```python
from build123d import *

# Parameters (mm, degrees)
SKETCH_1_R          = 17.5
EXTRUDE_1_DEPTH     = 9
SKETCH_2_R          = 1.3
CUT_EXTRUDE_1_DEPTH = 8
SKETCH_3_R          = 1.65
CUT_EXTRUDE_2_DEPTH = 9
SKETCH_4_R          = 7
CUT_EXTRUDE_3_DEPTH = 9
CHAMFER_1_SIZE      = 0.4
CHAMFER_1_SIZE2     = 1.098990968
SKETCH_5_R          = 3.2
CUT_EXTRUDE_4_DEPTH = 5


with BuildPart() as part:
    # 草图1 → 凸台-拉伸1 (new body)
    with BuildSketch(Plane.XY):
        Circle(SKETCH_1_R)
    extrude(amount=-EXTRUDE_1_DEPTH)

    # 草图2 → 切除-拉伸1 (cut)
    with BuildSketch(Plane.XY):
        with Locations((12.5, 0)):
            Circle(SKETCH_2_R)
        with Locations((0, -12.5)):
            Circle(SKETCH_2_R)
        with Locations((-12.5, 0)):
            Circle(SKETCH_2_R)
        with Locations((0, 12.5)):
            Circle(SKETCH_2_R)
    extrude(amount=-CUT_EXTRUDE_1_DEPTH, mode=Mode.SUBTRACT)

    # 草图3 → 切除-拉伸2 (cut)
    with BuildSketch(Plane.XY):
        with Locations((6.75, -11.691342951)):
            Circle(SKETCH_3_R)
        with Locations((-6.75, -11.691342951)):
            Circle(SKETCH_3_R)
        with Locations((-6.75, 11.691342951)):
            Circle(SKETCH_3_R)
        with Locations((6.75, 11.691342951)):
            Circle(SKETCH_3_R)
    extrude(amount=-CUT_EXTRUDE_2_DEPTH, mode=Mode.SUBTRACT)

    # 草图4 → 切除-拉伸3 (cut)
    with BuildSketch(Plane.XY):
        Circle(SKETCH_4_R)
    extrude(amount=-CUT_EXTRUDE_3_DEPTH, mode=Mode.SUBTRACT)

    # 倒角1
    chamfer_1_edges = [part.edges().sort_by_distance(p)[0] for p in [
        (-1.3, -12.5, 0),
        (-13.8, 0, 0),
        (-1.3, 12.5, 0),
        (11.2, 0, 0),
    ]]
    chamfer_1_side = [part.faces().sort_by_distance(p)[0] for p in [
        (-17.005025253, 0, 0),
    ]]
    chamfer(chamfer_1_edges, length=CHAMFER_1_SIZE, length2=CHAMFER_1_SIZE2, reference=chamfer_1_side[0])

    # 草图5 → 切除-拉伸4 (cut)
    with BuildSketch(Plane.XY):
        with Locations((-6.75, 11.691342951)):
            Circle(SKETCH_5_R)
        with Locations((6.75, 11.691342951)):
            Circle(SKETCH_5_R)
        with Locations((6.75, -11.691342951)):
            Circle(SKETCH_5_R)
        with Locations((-6.75, -11.691342951)):
            Circle(SKETCH_5_R)
    extrude(amount=-CUT_EXTRUDE_4_DEPTH, mode=Mode.SUBTRACT)


solid = part.part
```
Here's how the part is built. I have some questions about the finished solid (model axes, mm). A direction names the side the tool comes from. Give positions to 0.01 mm unless a question says otherwise; leave off trailing zeros. Loops run counter-clockwise (first coordinate to the right, second up) from the corner with the lowest first, then second, coordinate; pieces in that order, holes last. Notation, with made-up numbers: M 64,42 L 72,42 A10 ccw 72,56 Z; hole C 12,45 d6. An arc over 180 degrees is marked long. Put each result on its own line as item: value. Start each with the question number.
(1) I want a section at B-B on y = -12.5. Please give me the cut outline in (x, z), then the cut area to 3 significant figures.
(2) For faces 4 (the flat face through (8, 10, -5)), 5 (the cylindrical face through (6.39, 10.08, -6.97)), which set-ups out of +Z, -Z, +X, -X, +Y, -Y let a thin tool reach every point of the face, with its end or its side?
(3) I want a section at C-C on y = -5. Please give me the cut outline in (x, z).
(4) Will these pins go through, and if not, where does the flat tip stop? pin 1 Ø3 at (x, y) = (6.5, 11.5) entering from +Z; pin 2 Ø5 at (x, z) = (-12.5, -1.5) entering from -Y; pin 3 Ø2 at (x, z) = (13.5, -3) entering from +Y.
(5) I need wall thicknesses on line 1 along X through (y, z) = (-10, -1.25); line 2 along Y through (x, z) = (-0.5, -1.75); line 3 along Y through (x, z) = (-1, -5.5). Which ranges of each line are inside material? Lowest first, please. Write a range as [from, to].
(6) I want a section at A-A on x = 0. Please give me the cut outline in (y, z), then the cut area to 3 significant figures.
(7) I want a section at D-D on z = -3.25. State how many separate pieces and enclosed holes the cut face has, then the cut area to 3 significant figures.
(8) If we mould it in two halves opening along Y, with no side actions, what happens to faces 1 (the flat face through (12, 0, -8)), 2 (the flat face through (8, 0, 0)), 3 (the cylindrical face through (-7.11, 10.08, -6.97))? For each: +Y half, -Y half, draft (parallel to the pull), parting line (faces both ways), or undercut.
Answer block:
1. outline: M -12.25,-9 L -8.19,-9 L -8.19,-5 L -9.85,-5 L -9.85,0 L -12.25,0 Z; M -5.31,-9 L 5.31,-9 L 5.31,-5 L 3.65,-5 L 3.65,0 L 1.7,0 L 1.3,-1.1 L 1.3,-8 L -1.3,-8 L -1.3,-1.1 L -1.7,0 L -3.65,0 L -3.65,-5 L -5.31,-5 Z; M 8.19,-9 L 12.25,-9 L 12.25,0 L 9.85,0 L 9.85,-5 L 8.19,-5 Z
1. area: 114 mm^2
2. face 4: +Z
2. face 5: +Z, -Z
3. outline: M -16.77,-9 L -4.9,-9 L -4.9,0 L -16.77,0 Z; M 4.9,-9 L 16.77,-9 L 16.77,0 L 4.9,0 Z
4. pin 1: z = -5
4. pin 2: y = -14.36
4. pin 3: y = 12.25
5. line 1: [-14.36, -9.47], [-4.03, 4.03], [9.47, 14.36]
5. line 2: [-17.49, -13.7], [-11.3, -6.98], [6.98, 11.3], [13.7, 17.49]
5. line 3: [-17.47, -13.33], [-11.67, -6.93], [6.93, 11.67], [13.33, 17.47]
6. outline: M -17.5,-9 L -7,-9 L -7,0 L -10.8,0 L -11.2,-1.1 L -11.2,-8 L -13.8,-8 L -13.8,-1.1 L -14.2,0 L -17.5,0 Z; M 7,-9 L 17.5,-9 L 17.5,0 L 14.2,0 L 13.8,-1.1 L 13.8,-8 L 11.2,-8 L 11.2,-1.1 L 10.8,0 L 7,0 Z
6. area: 147 mm^2
7. separate pieces: 1
7. enclosed holes: 9
7. area: 658 mm^2
8. face 1: undercut
8. face 2: draft
8. face 3: undercut
